Autodesk Inventor part; units mm, degrees
ref_plane "Work Plane1" through (30.1625, 0, 0) normal (0, 0, -1) x (1, 0, 0)
ref_plane "YZ Plane" through (0, 0, 0) normal (1, 0, 0) x (0, 1, 0)
ref_plane "XZ Plane" through (0, 0, 0) normal (0, 1, 0) x (-1, 0, 0)
sketch "Sketch1" plane through (0, 0, 0) normal (0, 0, 1) x (1, 0, 0)
  line L0 (-3.3, 0) -> (50, 0)
  line L1 (50, 0) -> (50, 2.5)
  line L2 (50, 2.5) -> (1.6, 2.5)
  line L3 (1.6, 2.5) -> (1.1091, 2.2835)
  line L4 (1.1091, 2.2835) -> (0, 2.2835)
  line L5 (0, 2.2835) -> (0, 4.25)
  line L6 (-13.96, 0) -> (60.66, 0)
  line L7 (0, -0.85) -> (0, 5.1)
  line L8 (-3.3, 0) -> (-3.3, 3.9613)
  line L9 (0, 4.25) -> (-3.3, 3.9613)
  line L10 (1.6, 2.5) -> (0, 2.5) construction
  dimension "d0" = 50
  dimension "d1" = 48.4
  dimension "d2" = 0.4909
  dimension "d3" = 3.3
  dimension "d4" = 5
  dimension "d5" = 4.567
  dimension "d9" = 8.5
  dimension "d10" = 5
revolve "Body" add sketch "Sketch1" angle 360 about axis through (-3.3, 0, 0) along (1, 0, 0)
sketch "Sketch2" plane through (-3.3, 0, 0) normal (-1, 0, 0) x (0, 0, 1)
  circle A0 centre (0, 0) radius 4.25
  line L0 (0, 0) -> (0, 3.9613)
  line L1 (-4.25, 0.6) -> (4.25, 0.6)
  line L2 (4.25, 0.6) -> (4.25, -0.6)
  line L3 (4.25, -0.6) -> (-4.25, -0.6)
  line L4 (-4.25, -0.6) -> (-4.25, 0.6)
  line L5 (-4.25, 0) -> (4.25, 0) construction
  line L6 (0, 0.6) -> (0, -0.6) construction
  point P0 (0, 0)
  dimension "d11" = 1.2
  dimension "d12" = 8.5
fillet "Fillet1" radius 0.2 1 edges at (-3.3, -3.9613, 0)
extrude "Slot" cut sketch "Sketch2" against normal blind 1.3 contours A0 L3 L1 | L2 L3 A0 | A0 L1 L2 | A0 L4 L1 | L3 L4 A0
thread "Thread"
chamfer "Chamfer1" distance 0.433 distance2 0.4909 1 edges at (50, -2.5, 0) measured on face at (50, -0.4809, -0.0271)
ref_plane "Work Plane1" through (30.1625, 0, 0) normal (0, 0, -1) x (1, 0, 0)
equation "\"d11\" = SBR"
equation "\"d12\" = KOD"
equation "\"d14\" = RR"
equation "\"d19\" = STI"
equation "\"d15\" = GEL"
equation "\"d17\" = -0.5 * SPD + 0.5 * GD"
equation "\"d0\" = NLG"
equation "\"d1\" = GEL"
equation "\"d3\" = KOH"
equation "\"d4\" = GD"
equation "\"d5\" = BDM"
equation "\"d9\" = KOD"
equation "\"d10\" = KEWI"
equation "\"GD\" = 5"
equation "\"NLG\" = 50"
equation "\"GEL\" = 48.4"
equation "\"KOD\" = 8.5"
equation "\"KOH\" = 3.3"
equation "\"GAL\" = 0.61345 * PTC"
equation "\"SPD\" = 4.13397"
equation "\"BDM\" = 4.56699"
equation "\"GUL\" = 0.61345 * PTC"
equation "\"RR\" = 0.2"
equation "\"SBR\" = 1.2"
equation "\"STI\" = 1.3"
equation "\"KEWI\" = 5deg"
equation "\"PTC\" = 0.8"
equation "\"THREADDIA\" = 5"
equation "\"TOA\" = 30deg"
equation "\"NND\" = 5"
equation "\"GD1\" = THREADDIA - 1.2269 * PTC"
properties part number "DIN 84 - M5 x 50" material "Steel, Mild"
Part model, mm, in its own coordinate system. A direction names the side the tool comes from. Coordinates: 2 decimals unless noted, no trailing zeros. Order: outer loops, then holes, each group sorted by start corner. A loop starts at its lowest first (then second) coordinate and runs counter-clockwise, first axis right, second up.
(1) Slice it at B-B, the plane z = 0. Write the cut outline in (x, y), and give its area (3 significant figures).
Check sheet entries:
outline: (-3.3, -3.78) arc R0.2 ccw to (-3.12, -3.98) - (0, -4.25) - (0, -2.28) - (1.11, -2.28) - (1.6, -2.5) - (49.51, -2.5) - (50, -2.07) - (50, 2.07) - (49.51, 2.5) - (1.6, 2.5) - (1.11, 2.28) - (0, 2.28) - (0, 4.25) - (-3.12, 3.98) arc R0.2 ccw to (-3.3, 3.78) - (-3.3, 0.6) - (-2, 0.6) - (-2, -0.6) - (-3.3, -0.6) - close
area: 275 mm2
(2) Slice it at A-A, the plane y = 0. Write the cut outline in (x, z), and give its area (3 significant figures).
Check sheet entries:
outline: (-2, -4.08) - (0, -4.25) - (0, -2.28) - (1.11, -2.28) - (1.6, -2.5) - (49.51, -2.5) - (50, -2.07) - (50, 2.07) - (49.51, 2.5) - (1.6, 2.5) - (1.11, 2.28) - (0, 2.28) - (0, 4.25) - (-2, 4.08) - close
area: 266 mm2
(3) Tool access for faces 5 (the face through (-3.3, 2, 0)), 6 (the face through (-3, 0.6, 0)): list every direction of +Z, -Z, +X, -X, +Y, -Y with a clear straight run to the whole face (end or side of a thin tool).
Check sheet entries:
face 5: +Z, -Z, -X, +Y, -Y
face 6: +Z, -Z, -X
(4) Pin check, flat tips, straight feed: pin 1 Ø2 at (x, y) = (18, 1.5) entering from -Z; pin 2 Ø3 at (x, z) = (38.5, -3) entering from +Y; pin 3 Ø2 at (x, z) = (40.5, -3) entering from -Y. Stop position of each tip, or through.
Check sheet entries:
pin 1: stops at z = -2.45
pin 2: stops at y = 2
pin 3: stops at y = -1.5
(5) Pull direction X, two halves, no side cores. Call faces 1 (the face through (25.22, -0.54, 2.44)), 2 (the face through (-1.883, -0.886, -3.988)), 3 (the face through (50, 0, 0)), 4 (the face through (0.547, 2.178, -0.686)): pulls with the +X half, pulls with the -X half, needs draft (parallel to the pull), parting line crosses it, or undercut.
Check sheet entries:
face 1: needs draft
face 2: pulls with the -X half
face 3: pulls with the +X half
face 4: undercut
(6) Probe L1, parallel to X at y = 2.25, z = 0.75; L2, parallel to Y at x = 44, z = -1; L3, parallel to X at y = -2.75, z = 2. List the from-to ranges inside material, lowest first.
Check sheet entries:
L1: x = -3.3 to 0, 1.31 to 49.65
L2: y = -2.29 to 2.29
L3: x = -3.3 to 0
(7) Slice it at C-C, the plane x = 24. Write the cut outline in (y, z).
Check sheet entries:
outline: circle Ø5 at (0, 0)
